For this review, use the dimensioned drawing (mm, ordinates from the lowest corner) and the shaded views. A direction names the side the tool comes from. Coordinates: 2 decimals unless noted, no trailing zeros. Write each loop counter-clockwise with the first axis right and the second up, starting at its lowest first coordinate (ties: lowest second). Pieces come first, ordered by that corner, then holes. Notation, with made-up numbers: (73, -23.5) -> (105, -23.5) arc R29 cw to (105, 7.5) -> close; hole circle Ø6 at (57.25, -38). An arc over 180 degrees is marked (long way). Return JSON: item names as keys, results as strings. Group by question number.
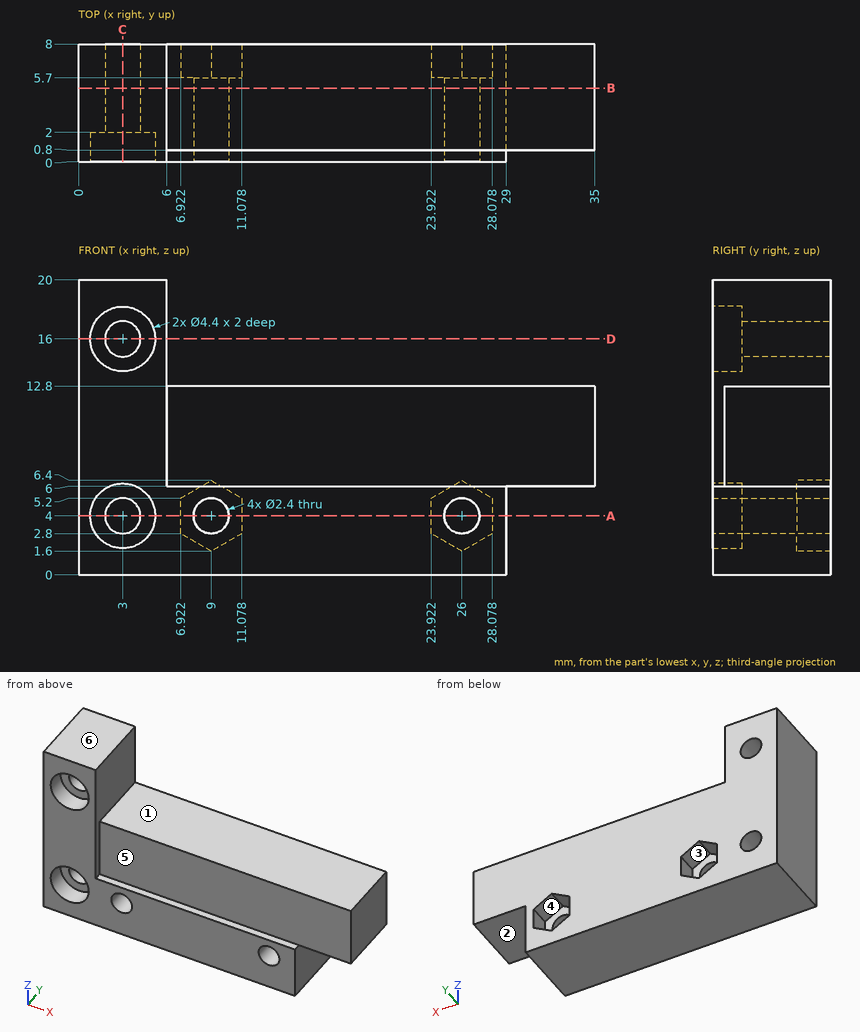
Q1. We need section C-C on x = 3. Write out the cut boundary in (y, z).
Q2. The part is to be moulded in two halves that separate along Z. For the marked faces 4, 5 and 6, say which applies: +Z half, -Z half, draft (parallel to the pull), parting line (faces both ways), or undercut.
Q3. We need section B-B on y = 5. Write out the cut boundary in (x, z).
Q4. We need section A-A on z = 4. Write out the cut boundary in (x, y).
Q5. For the marked faces 1, 2 and 3, list the 3-axis set-ups (+Z, -Z, +X, -X, +Y, -Y) from which the entire face can be reached by the end or side of a thin tool; tool diameter is ignored.
Q6. For P1, Ø2.5, axis at y = 7, z = 4, coming from the +X side; P2, Ø3.5, axis at x = 15.5, z = 10, coming from the -Y side; P3, Ø1, axis at x = 18.5, y = 7, coming from the +Z side, all flat-tipped, find the tip position at first contact; note any pin that passes through.
Q7. We need section D-D on z = 16. Write out the cut boundary in (x, y), plus the area to 3 significant figures.
Q8. Wall thickness on L1, parallel to Z at x = 3, y = 3.35; L2, parallel to X at y = 3.5, z = 4; L3, parallel to X at y = 1.65, z = 4: over which ranges is each line inside the solid? List them lowest first.
Findings below:
{
 "1": {"outline": "(0, 0) -> (8, 0) -> (8, 2.8) -> (2, 2.8) -> (2, 1.8) -> (0, 1.8) -> close; (0, 6.2) -> (2, 6.2) -> (2, 5.2) -> (8, 5.2) -> (8, 14.8) -> (2, 14.8) -> (2, 13.8) -> (0, 13.8) -> close; (0, 18.2) -> (2, 18.2) -> (2, 17.2) -> (8, 17.2) -> (8, 20) -> (0, 20) -> close"},
 "2": {"face 4": "undercut", "face 5": "draft", "face 6": "+Z half"},
 "3": {"outline": "(0, 0) -> (29, 0) -> (29, 6) -> (35, 6) -> (35, 12.8) -> (6, 12.8) -> (6, 20) -> (0, 20) -> close; hole circle Ø2.4 at (3, 4); hole circle Ø2.4 at (3, 16); hole circle Ø2.4 at (9, 4); hole circle Ø2.4 at (26, 4)"},
 "4": {"outline": "(0, 0) -> (0.8, 0) -> (0.8, 2) -> (1.8, 2) -> (1.8, 8) -> (0, 8) -> close; (4.2, 2) -> (5.2, 2) -> (5.2, 0) -> (7.8, 0) -> (7.8, 5.7) -> (6.92, 5.7) -> (6.92, 8) -> (4.2, 8) -> close; (10.2, 0) -> (24.8, 0) -> (24.8, 5.7) -> (23.92, 5.7) -> (23.92, 8) -> (11.08, 8) -> (11.08, 5.7) -> (10.2, 5.7) -> close; (27.2, 0) -> (29, 0) -> (29, 8) -> (28.08, 8) -> (28.08, 5.7) -> (27.2, 5.7) -> close"},
 "5": {"face 1": "+Z, +X, +Y, -Y", "face 2": "-Z, +X, +Y, -Y", "face 3": "+Y"},
 "6": {"P1": "stops at x = 29", "P2": "stops at y = 0.8", "P3": "stops at z = 12.8"},
 "7": {"outline": "(0, 0) -> (0.8, 0) -> (0.8, 2) -> (1.8, 2) -> (1.8, 8) -> (0, 8) -> close; (4.2, 2) -> (5.2, 2) -> (5.2, 0) -> (6, 0) -> (6, 8) -> (4.2, 8) -> close", "area": "24.8 mm^2"},
 "8": {"L1": "z = 0 to 2.8, 5.2 to 14.8, 17.2 to 20", "L2": "x = 0 to 1.8, 4.2 to 7.8, 10.2 to 24.8, 27.2 to 29", "L3": "x = 0 to 0.8, 5.2 to 7.8, 10.2 to 24.8, 27.2 to 29"}
}
